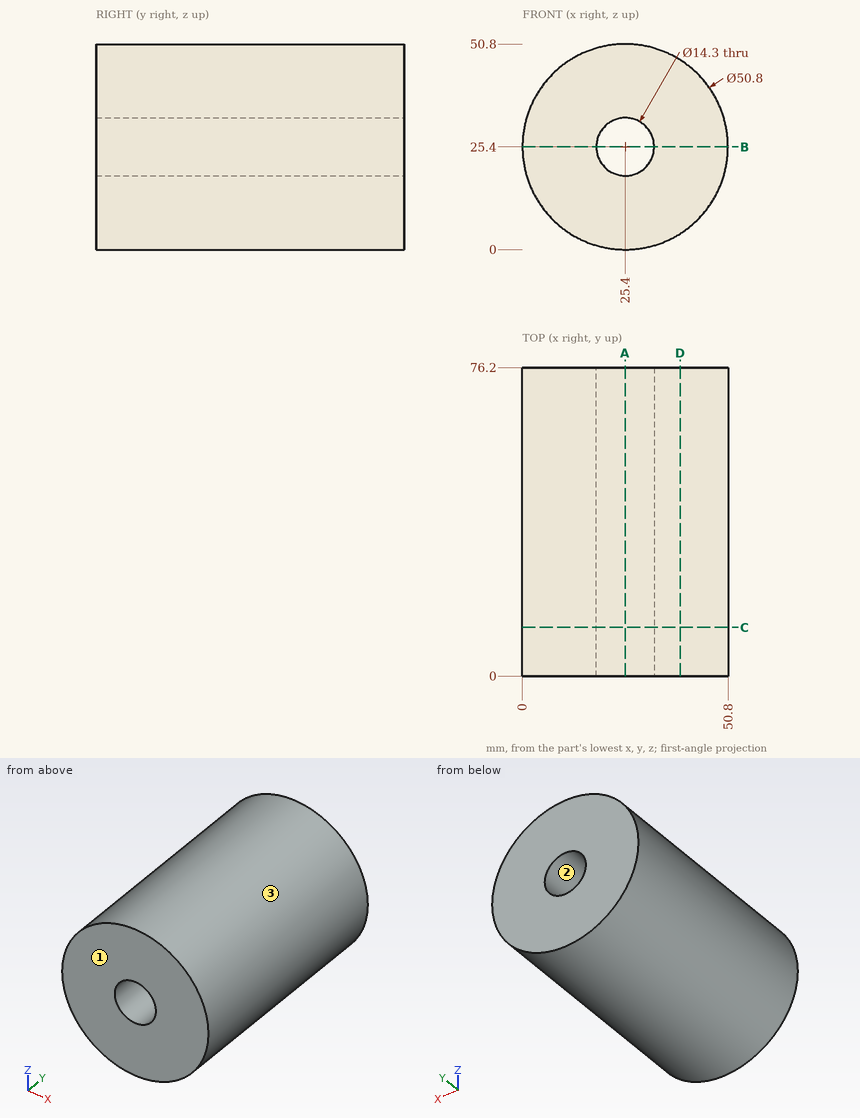
Geometry check sheet. Reference: drawing and pictorial views, mm from the part's lowest x, y, z. Round coordinates to 2 decimals unless told otherwise and drop trailing zeros. Order: outer loops, then holes, each group sorted by start corner. A loop starts at its lowest first (then second) coordinate and runs counter-clockwise, first axis right, second up. Notation, with made-up numbers: (-24.75, 62.5) - (27.25, 62.5) arc R6 cw to (27.25, 66.5) - close; hole circle Ø1 at (20.25, 57). An arc over 180 degrees is marked (long way). One line per question, with ' | ' between items. Start each with the question number.
(1) Sectioned sample at B-B on z = 25.4. Record the cut outline in (x, y), and give its area (3 significant figures).
(2) Thickness scan on L1, parallel to Z at x = 25.4, y = 46.5; L2, parallel to X at y = 32, z = 23 (1 decimal); L3, parallel to Z at x = 27.5, y = 9.5 (1 decimal). Record the ranges inside material, lowest first. Write a range as [from, to].
(3) Sectioned sample at C-C on y = 12. Record the cut outline in (x, z), and give its area (3 significant figures).
(4) Depth check by flat-ended pin: pin 1 Ø4 at (x, y) = (35, 25.5) entering from +Z; pin 2 Ø6 at (x, y) = (21, 61.5) entering from -Z; pin 3 Ø1.5 at (y, z) = (25, 21.5) entering from -X; pin 4 Ø13 at (x, z) = (25.4, 25.4) entering from +Y. Enter the tip coordinate at first touch or a pass-through.
(5) Release check for a two-part mould opening along X. For the marked faces 1, 2 and 3 record: released by +X, released by -X, zero draft, split by the parting line, or undercut.
(6) Sectioned sample at A-A on x = 25.4. Record the cut outline in (y, z).
(7) Sectioned sample at D-D on x = 39. Record the cut outline in (y, z).
Conclusion:
1) outline: (0, 0) - (18.25, 0) - (18.25, 76.2) - (0, 76.2) - close; (32.55, 0) - (50.8, 0) - (50.8, 76.2) - (32.55, 76.2) - close | area: 2,780 mm2
2) L1: z = [0, 18.25], [32.55, 50.8] | L2: x = [0.1, 18.7], [32.1, 50.7] | L3: z = [0.1, 18.6], [32.2, 50.7]
3) outline: circle Ø50.8 at (25.4, 25.4); hole circle Ø14.3 at (25.4, 25.4) | area: 1,870 mm2
4) pin 1: stops at z = 49.64 | pin 2: stops at z = 0.04 | pin 3: stops at x = 0.2 | pin 4: passes through
5) face 1: zero draft | face 2: undercut | face 3: split by the parting line
6) outline: (0, 0) - (76.2, 0) - (76.2, 18.25) - (0, 18.25) - close; (0, 32.55) - (76.2, 32.55) - (76.2, 50.8) - (0, 50.8) - close
7) outline: (0, 3.95) - (76.2, 3.95) - (76.2, 46.85) - (0, 46.85) - close
